Geometry: see drawing. Coordinates: mm, zero at the bounding-box minimum. A direction names the side the tool comes from. Round coordinates to 2 decimals unless told otherwise and drop trailing zeros. Order: outer loops, then holes, each group sorted by start corner. A loop starts at its lowest first (then second) coordinate and runs counter-clockwise, first axis right, second up. Notation, with made-up numbers: (-25, 77) - (-10, 77) arc R36 ccw to (-10, 111) - close; hole circle Ø1 at (63, -34). An arc over 180 degrees is marked (long way). Put each result on its own line as item: value. Start each with the question number.
1) Section B-B on y = 17.25. Output: boundary loops of the cut face in (x, z), then the cut area to 3 significant figures.
2) Contact query for flat-ended pins moving along their axis: P1, Ø1.5, axis at x = 16, z = 20, coming from the +Y side; P2, Ø2, axis at x = 13.5, z = 32, coming from the -Y side; P3, Ø14.5, axis at y = 17.25, z = 32.5, coming from the -X side. Output: stop coordinate, or through.
3) Section C-C on z = 10. Output: boundary loops of the cut face in (x, y), then the cut area to 3 significant figures.
4) Section D-D on y = 35. Output: boundary loops of the cut face in (x, z), then the cut area to 3 significant figures.
5) Section A-A on z = 32.5. Output: boundary loops of the cut face in (x, y).
6) Line query: probe 1 along Y at (x, z) = (66, 32); probe 2 along Z at (x, y) = (67.9, 17.25); probe 3 along Y at (x, z) = (17.5, 20). Output: solid intervals per line, ascending. Write a range as [from, to].
7) Access query for the marked faces 1 and 2. Directions: +Z, -Z, +X, -X, +Y, -Y. A direction counts if a zero-diameter tool reaches every point of the face in a straight line with its end or side. Return the directions, or none.
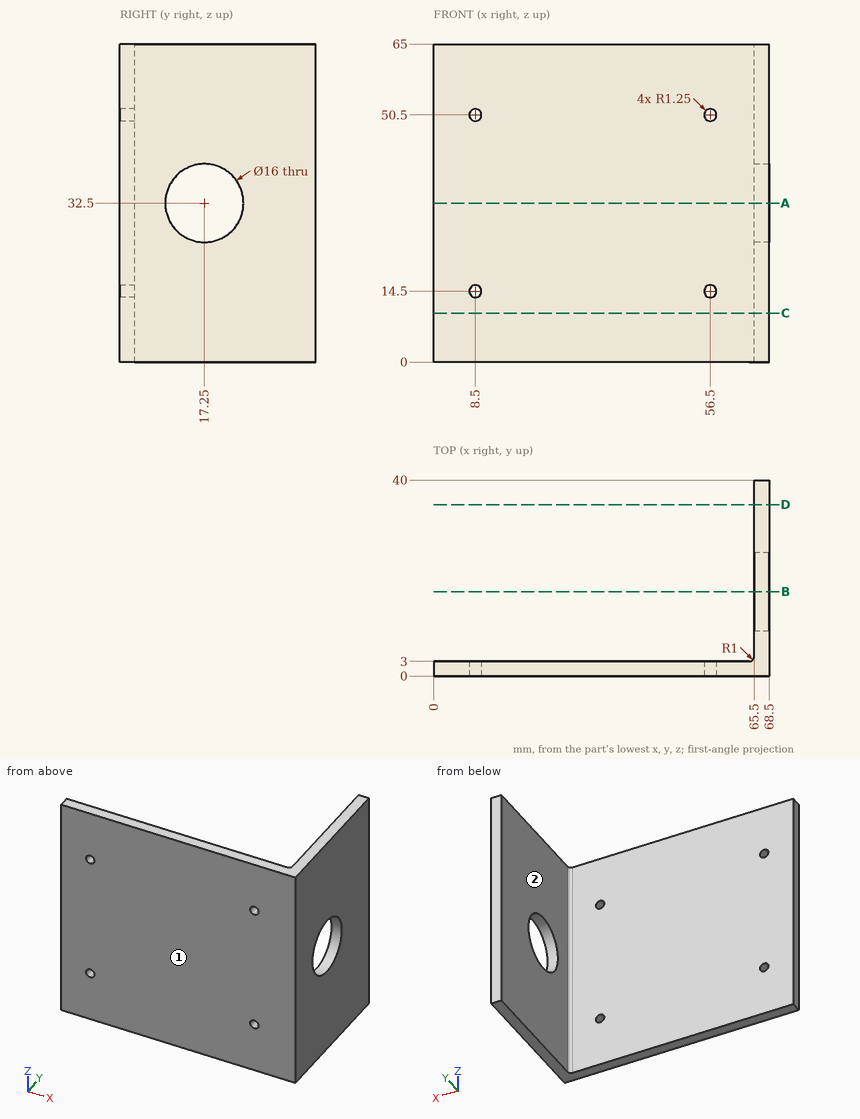
Answer sheet:
1. outline: (65.5, 0) - (68.5, 0) - (68.5, 24.5) - (65.5, 24.5) - close; (65.5, 40.5) - (68.5, 40.5) - (68.5, 65) - (65.5, 65) - close
1. area: 147 mm^2
2. P1: y = 3
2. P2: y = 0
2. P3: through
3. outline: (0, 0) - (68.5, 0) - (68.5, 40) - (65.5, 40) - (65.5, 4) arc R1 cw to (64.5, 3) - (0, 3) - close
3. area: 317 mm^2
4. outline: (65.5, 0) - (68.5, 0) - (68.5, 65) - (65.5, 65) - close
4. area: 195 mm^2
5. outline: (0, 0) - (68.5, 0) - (68.5, 9.25) - (65.5, 9.25) - (65.5, 4) arc R1 cw to (64.5, 3) - (0, 3) - close; (65.5, 25.25) - (68.5, 25.25) - (68.5, 40) - (65.5, 40) - close
6. probe 1: [0, 9.27], [25.23, 40]
6. probe 2: [0, 24.5], [40.5, 65]
6. probe 3: [0, 3]
7. face 1: +Z, -Z, +X, -X, -Y
7. face 2: +Z, -Z, -X, +Y
